```python
from build123d import *

# Parameters (mm, degrees)
EXTRUDE_1_DEPTH     = 21
EXTRUDE_2_DEPTH     = 5
SKETCH_5_R          = 5.2
CUT_EXTRUDE_1_DEPTH = 121.108284477


with BuildPart() as part:
    # 草图1 → 凸台-拉伸1 (new, symmetric)
    with BuildSketch(Plane.XY):
        Polygon((-88, 0), (0, 0), (0, 88), (-9, 88), (-9, 9), (-88, 9), align=None)
    extrude(amount=EXTRUDE_1_DEPTH, both=True)

    # 草图4 → 凸台-拉伸2 (add)
    with BuildSketch(Plane(origin=(0, 0, -21), x_dir=(-1, 0, 0), z_dir=(0, 0, -1))):
        with BuildLine():
            Line((88, 9), (88, 12.5))
            ThreePointArc((88, 12.5), (87.121320344, 14.621320344), (85, 15.5))
            Line((85, 15.5), (82, 15.5))
            Line((82, 15.5), (15.5, 82))
            Line((15.5, 82), (15.5, 85))
            ThreePointArc((15.5, 85), (14.621320344, 87.121320344), (12.5, 88))
            Line((12.5, 88), (9, 88))
            Line((9, 88), (9, 9))
            Line((9, 9), (88, 9))
        make_face()
    extrude(amount=-EXTRUDE_2_DEPTH)

    # 草图5 → 切除-拉伸1 (cut, through all)
    with BuildSketch(Plane(origin=(0, 9, 0), x_dir=(1, 0, 0), z_dir=(0, 1, 0))):
        with Locations(Location((-67.5, 0, 0), (0, 0, 270))):
            Circle(SKETCH_5_R)
        with BuildLine():
            Line((-45, 5.2), (-22.5, 5.2))
            ThreePointArc((-22.5, 5.2), (-17.3, 0), (-22.5, -5.2))
            Line((-22.5, -5.2), (-45, -5.2))
            ThreePointArc((-45, -5.2), (-50.2, 0), (-45, 5.2))
        make_face()
    cut_extrude_1 = extrude(amount=-CUT_EXTRUDE_1_DEPTH, mode=Mode.SUBTRACT)

    # 镜向1: 切除-拉伸1 across plane
    add(cut_extrude_1.mirror(Plane(origin=(0, 0, 0), x_dir=(0, 0, 1), z_dir=(-0.7071067811865477, -0.7071067811865475, 0))), mode=Mode.SUBTRACT)


solid = part.part
```
Geometry: final body of the model. Coordinates: model frame, mm. A direction names the side the tool comes from. Coordinates: 2 decimals unless noted, no trailing zeros. Write each loop counter-clockwise with the first axis right and the second up, starting at its lowest first coordinate (ties: lowest second). Pieces come first, ordered by that corner, then holes. Notation, with made-up numbers: M 86,82 L 125,82 A14 cw 125,100 Z; hole C 45.5,70.5 d9. An arc over 180 degrees is marked long. Use CSV: the item, a comma, the result in double quotes. Start each with the question number.
1. Ray query, probe 1 along X at (y, z) = (3, 0); probe 2 along Y at (x, z) = (-3, 0); probe 3 along Z at (x, y) = (-7, 67). Return the intervals inside material, ascending.
2. Cut plane C-C on z = 0. Return the cut outline in (x, y), plus the area to 3 significant figures.
3. Cut plane D-D on z = -8.5. Return the cut outline in (x, y), plus the area to 3 significant figures.
4. Reachability of faces 4 (the face through (-39, 40, -16)), 5 (the face through (-34, 5, -5.2)), 6 (the face through (-4.6, 17.3, -0.1)) from +Z, -Z, +X, -X, +Y, -Y: full face, straight path, thin tool, end or side. Return the list, or none.
5. First-contact query: P1, Ø2.5, axis at x = -83.5, z = -19.5, coming from the +Y side; P2, Ø12, axis at x = -26, y = 27.5, coming from the +Z side; P3, Ø1.5, axis at y = 83, z = -18, coming from the -X side. Flat tips, straight axial feed; report the tip coordinate or a pass-through.
6. Cut plane A-A on x = -67.5. Return the cut outline in (y, z), plus the area to 3 significant figures.
7. Mould query, pull axis Y, two halves, no side actions, for faces 1 (the face through (-5, 88, 0)), 2 (the face through (-5, 34, 5.2)), 3 (the face through (-62.344, 4.563, -0.677)). Classes: pulls with the +Y half, pulls with the -Y half, needs draft (parallel to the pull), parting line crosses it, or undercut.
8. Cut plane B-B on y = 20.5. Return the cut outline in (x, z).
Entries:
1,probe 1,"-88 to -72.7, -62.3 to -50.2, -17.3 to 0"
1,probe 2,"0 to 17.3, 50.2 to 62.3, 72.7 to 88"
1,probe 3,"-21 to -5.18, 5.18 to 21"
2,outline,"M -88,0 L -72.7,0 L -72.7,9 L -88,9 Z; M -62.3,0 L -50.2,0 L -50.2,9 L -62.3,9 Z; M -17.3,0 L 0,0 L 0,17.3 L -9,17.3 L -9,9 L -17.3,9 Z; M -9,50.2 L 0,50.2 L 0,62.3 L -9,62.3 Z; M -9,72.7 L 0,72.7 L 0,88 L -9,88 Z"
2,area,"724 mm²"
3,outline,"M -88,0 L 0,0 L 0,88 L -9,88 L -9,9 L -88,9 Z"
3,area,"1,500 mm²"
4,face 4,"+Z, -X, +Y"
4,face 5,"+Y, -Y"
4,face 6,"+X, -X"
5,P1,"y = 15.5"
5,P2,"z = -16"
5,P3,"x = -15.5"
6,outline,"M 0,-21 L 30,-21 L 30,-16 L 9,-16 L 9,-5.2 L 0,-5.2 Z; M 0,5.2 L 9,5.2 L 9,21 L 0,21 Z"
6,area,"389 mm²"
7,face 1,"pulls with the +Y half"
7,face 2,"undercut"
7,face 3,"needs draft"
8,outline,"M -77,-21 L 0,-21 L 0,-4.8 L -9,-4.8 L -9,-16 L -77,-16 Z; M -9,4.8 L 0,4.8 L 0,21 L -9,21 Z"
